Geometry: final body of the model. Coordinates: model frame, mm. A direction names the side the tool comes from. Coordinates: 2 decimals unless noted, no trailing zeros. Loops run counter-clockwise (first coordinate to the right, second up) from the corner with the lowest first, then second, coordinate; pieces in that order, holes last. Notation, with made-up numbers: (-1.5, 50.25) -> (28.5, 50.25) arc R25 ccw to (28.5, 74.25) -> close; hole circle Ø9 at (36, 34.25). An arc over 180 degrees is marked (long way). One line per item, written item: value. Start each with the question number.
from build123d import *

# Parameters (mm, degrees)
SKETCH_1_W              = 180
SKETCH_1_H              = 125
EXTRUDE_1_DEPTH         = 25
SKETCH_2_W              = 130
SKETCH_2_H              = 125
EXTRUDE_2_DEPTH         = 39
SKETCH_3_R              = 10
CUT_EXTRUDE_1_DEPTH     = 12
SKETCH_4_R              = 10
CUT_EXTRUDE_2_DEPTH     = 12
SKETCH_6_R              = 10
CUT_EXTRUDE_3_DEPTH     = 12
SKETCH_7_R              = 10
CUT_EXTRUDE_4_DEPTH     = 12
SKETCH_9_R              = 6.5
CUT_EXTRUDE_6_DEPTH     = 13
SKETCH_10_R             = 6.5
CUT_EXTRUDE_7_DEPTH     = 13
SKETCH_11_R             = 6.5
CUT_EXTRUDE_8_DEPTH     = 13
SKETCH_12_R             = 6.5
CUT_EXTRUDE_9_DEPTH     = 13
HOLE_WIZARD_M12_1_D     = 10.2
HOLE_WIZARD_M12_1_DEPTH = 25
HOLE_WIZARD_M12_1_TIP   = 3.064389157
HOLE_WIZARD_M12_2_D     = 10.2
HOLE_WIZARD_M12_2_DEPTH = 25
HOLE_WIZARD_M12_2_TIP   = 3.064389157
HOLE_WIZARD_M12_3_D     = 10.2
HOLE_WIZARD_M12_3_DEPTH = 25
HOLE_WIZARD_M12_3_TIP   = 3.064389157
HOLE_WIZARD_M12_4_D     = 10.2
HOLE_WIZARD_M12_4_DEPTH = 25
HOLE_WIZARD_M12_4_TIP   = 3.064389157
SKETCH_23_R             = 10.65
CUT_EXTRUDE_12_DEPTH    = 2
HOLE_WIZARD_M12_5_D     = 10.2
HOLE_WIZARD_M12_5_DEPTH = 25
HOLE_WIZARD_M12_5_TIP   = 3.064389157
HOLE_WIZARD_M12_6_D     = 10.2
HOLE_WIZARD_M12_6_DEPTH = 25
HOLE_WIZARD_M12_6_TIP   = 3.064389157
HOLE_WIZARD_M12_7_D     = 10.2
HOLE_WIZARD_M12_7_DEPTH = 25
HOLE_WIZARD_M12_7_TIP   = 3.064389157
FILLET_7_R              = 1
FILLET_8_R              = 1
FILLET_10_R             = 1
SKETCH_33_R             = 10.65
CUT_EXTRUDE_13_DEPTH    = 1.97
SKETCH_36_R             = 11.5
CUT_EXTRUDE_15_DEPTH    = 2
M16X1_5_2_D             = 14.5
M16X1_5_2_DEPTH         = 14
M16X1_5_2_TIP           = 4.356239488
SKETCH_38_R             = 6
CUT_EXTRUDE_16_DEPTH    = 63.03
MM_1_D                  = 12
MM_1_DEPTH              = 33.63
MM_1_TIP                = 3.605163714
SKETCH_41_R             = 11.5
CUT_EXTRUDE_17_DEPTH    = 2
SKETCH_39_R             = 10.65
CUT_EXTRUDE_18_DEPTH    = 1.97
CUT_EXTRUDE_19_REACH    = 125
SKETCH_42_R             = 6
M16X1_5_3_D             = 14.5
M16X1_5_3_DEPTH         = 14
M16X1_5_3_TIP           = 4.356239488
FILLET_11_R             = 1


with BuildPart() as part:
    # 草图1 → 凸台-拉伸1 (new body)
    with BuildSketch(Plane(origin=(0, 0, 0), x_dir=(1, 0, 0), z_dir=(0, 1, 0))):
        Rectangle(SKETCH_1_W, SKETCH_1_H)
    extrude(amount=EXTRUDE_1_DEPTH)

    # 草图2 → 凸台-拉伸2 (add)
    with BuildSketch(Plane(origin=(0, 25, 0), x_dir=(1, 0, 0), z_dir=(0, 1, 0))):
        Rectangle(SKETCH_2_W, SKETCH_2_H)
    extrude(amount=EXTRUDE_2_DEPTH)

    # 草图3 → 切除-拉伸1 (cut)
    with BuildSketch(Plane(origin=(0, 25, 0), x_dir=(1, 0, 0), z_dir=(0, 1, 0))):
        with Locations((-78, 44.5)):
            Circle(SKETCH_3_R)
    extrude(amount=-CUT_EXTRUDE_1_DEPTH, mode=Mode.SUBTRACT)

    # 草图4 → 切除-拉伸2 (cut)
    with BuildSketch(Plane(origin=(0, 25, 0), x_dir=(1, 0, 0), z_dir=(0, 1, 0))):
        with Locations((78, 44.5)):
            Circle(SKETCH_4_R)
    extrude(amount=-CUT_EXTRUDE_2_DEPTH, mode=Mode.SUBTRACT)

    # 草图6 → 切除-拉伸3 (cut)
    with BuildSketch(Plane(origin=(0, 25, 0), x_dir=(1, 0, 0), z_dir=(0, 1, 0))):
        with Locations((-78, -44.5)):
            Circle(SKETCH_6_R)
    extrude(amount=-CUT_EXTRUDE_3_DEPTH, mode=Mode.SUBTRACT)

    # 草图7 → 切除-拉伸4 (cut)
    with BuildSketch(Plane(origin=(0, 25, 0), x_dir=(1, 0, 0), z_dir=(0, 1, 0))):
        with Locations((78, -44.5)):
            Circle(SKETCH_7_R)
    extrude(amount=-CUT_EXTRUDE_4_DEPTH, mode=Mode.SUBTRACT)

    # 草图9 → 切除-拉伸6 (cut)
    with BuildSketch(Plane(origin=(0, 13, 0), x_dir=(1, 0, 0), z_dir=(0, 1, 0))):
        with Locations((-78, -44.5)):
            Circle(SKETCH_9_R)
    extrude(amount=-CUT_EXTRUDE_6_DEPTH, mode=Mode.SUBTRACT)

    # 草图10 → 切除-拉伸7 (cut)
    with BuildSketch(Plane(origin=(0, 13, 0), x_dir=(1, 0, 0), z_dir=(0, 1, 0))):
        with Locations((-78, 44.5)):
            Circle(SKETCH_10_R)
    extrude(amount=-CUT_EXTRUDE_7_DEPTH, mode=Mode.SUBTRACT)

    # 草图11 → 切除-拉伸8 (cut)
    with BuildSketch(Plane(origin=(0, 13, 0), x_dir=(1, 0, 0), z_dir=(0, 1, 0))):
        with Locations((78, 44.5)):
            Circle(SKETCH_11_R)
    extrude(amount=-CUT_EXTRUDE_8_DEPTH, mode=Mode.SUBTRACT)

    # 草图12 → 切除-拉伸9 (cut)
    with BuildSketch(Plane(origin=(0, 13, 0), x_dir=(1, 0, 0), z_dir=(0, 1, 0))):
        with Locations((78, -44.5)):
            Circle(SKETCH_12_R)
    extrude(amount=-CUT_EXTRUDE_9_DEPTH, mode=Mode.SUBTRACT)

    # M12 螺纹孔1
    with Locations(Plane(origin=(0, 64, 0), x_dir=(1, 0, 0), z_dir=(0, 1, 0))):
        with Locations((-55, 52.5)):
            Hole(HOLE_WIZARD_M12_1_D / 2, depth=HOLE_WIZARD_M12_1_DEPTH)
            with Locations((0, 0, -(HOLE_WIZARD_M12_1_DEPTH + HOLE_WIZARD_M12_1_TIP / 2))):  # 118° drill point
                Cone(0, HOLE_WIZARD_M12_1_D / 2, HOLE_WIZARD_M12_1_TIP, mode=Mode.SUBTRACT)

    # M12 螺纹孔2
    with Locations(Plane(origin=(55, 64, -52.5), x_dir=(0, 0, 1), z_dir=(0, 1, 0))):
        with Locations((0, 0)):
            Hole(HOLE_WIZARD_M12_2_D / 2, depth=HOLE_WIZARD_M12_2_DEPTH)
            with Locations((0, 0, -(HOLE_WIZARD_M12_2_DEPTH + HOLE_WIZARD_M12_2_TIP / 2))):  # 118° drill point
                Cone(0, HOLE_WIZARD_M12_2_D / 2, HOLE_WIZARD_M12_2_TIP, mode=Mode.SUBTRACT)

    # M12 螺纹孔3
    with Locations(Plane(origin=(-55, 64, 52.5), x_dir=(0, 0, 1), z_dir=(0, 1, 0))):
        with Locations((0, 0)):
            Hole(HOLE_WIZARD_M12_3_D / 2, depth=HOLE_WIZARD_M12_3_DEPTH)
            with Locations((0, 0, -(HOLE_WIZARD_M12_3_DEPTH + HOLE_WIZARD_M12_3_TIP / 2))):  # 118° drill point
                Cone(0, HOLE_WIZARD_M12_3_D / 2, HOLE_WIZARD_M12_3_TIP, mode=Mode.SUBTRACT)

    # M12 螺纹孔4
    with Locations(Plane(origin=(55, 64, 52.5), x_dir=(0, 0, 1), z_dir=(0, 1, 0))):
        with Locations((0, 0)):
            Hole(HOLE_WIZARD_M12_4_D / 2, depth=HOLE_WIZARD_M12_4_DEPTH)
            with Locations((0, 0, -(HOLE_WIZARD_M12_4_DEPTH + HOLE_WIZARD_M12_4_TIP / 2))):  # 118° drill point
                Cone(0, HOLE_WIZARD_M12_4_D / 2, HOLE_WIZARD_M12_4_TIP, mode=Mode.SUBTRACT)

    # 草图23 → 切除-拉伸12 (cut)
    with BuildSketch(Plane.XZ):
        with Locations((-35, -27.5)):
            Circle(SKETCH_23_R)
    extrude(amount=-CUT_EXTRUDE_12_DEPTH, mode=Mode.SUBTRACT)

    # M12 螺纹孔5
    with Locations(Plane(origin=(55, 64, -52.5), x_dir=(0, 0, 1), z_dir=(0, 1, 0))):
        with Locations((0, 0)):
            Hole(HOLE_WIZARD_M12_5_D / 2, depth=HOLE_WIZARD_M12_5_DEPTH)
            with Locations((0, 0, -(HOLE_WIZARD_M12_5_DEPTH + HOLE_WIZARD_M12_5_TIP / 2))):  # 118° drill point
                Cone(0, HOLE_WIZARD_M12_5_D / 2, HOLE_WIZARD_M12_5_TIP, mode=Mode.SUBTRACT)

    # M12 螺纹孔6
    with Locations(Plane(origin=(-55, 64, 52.5), x_dir=(0, 0, 1), z_dir=(0, 1, 0))):
        with Locations((0, 0)):
            Hole(HOLE_WIZARD_M12_6_D / 2, depth=HOLE_WIZARD_M12_6_DEPTH)
            with Locations((0, 0, -(HOLE_WIZARD_M12_6_DEPTH + HOLE_WIZARD_M12_6_TIP / 2))):  # 118° drill point
                Cone(0, HOLE_WIZARD_M12_6_D / 2, HOLE_WIZARD_M12_6_TIP, mode=Mode.SUBTRACT)

    # M12 螺纹孔7
    with Locations(Plane(origin=(55, 64, 52.5), x_dir=(0, 0, 1), z_dir=(0, 1, 0))):
        with Locations((0, 0)):
            Hole(HOLE_WIZARD_M12_7_D / 2, depth=HOLE_WIZARD_M12_7_DEPTH)
            with Locations((0, 0, -(HOLE_WIZARD_M12_7_DEPTH + HOLE_WIZARD_M12_7_TIP / 2))):  # 118° drill point
                Cone(0, HOLE_WIZARD_M12_7_D / 2, HOLE_WIZARD_M12_7_TIP, mode=Mode.SUBTRACT)

    # 圆角7
    fillet_7_edges = [part.edges().sort_by_distance(p)[0] for p in [
        (-90, 25, 0),
    ]]
    fillet(fillet_7_edges, radius=FILLET_7_R)

    # 圆角8
    fillet_8_edges = [part.edges().sort_by_distance(p)[0] for p in [
        (-65, 25, 0),
    ]]
    fillet(fillet_8_edges, radius=FILLET_8_R)

    # 圆角10
    fillet_10_edges = [part.edges().sort_by_distance(p)[0] for p in [
        (65, 25, 0),
    ]]
    fillet(fillet_10_edges, radius=FILLET_10_R)

    # 草图33 → 切除-拉伸13 (cut)
    with BuildSketch(Plane(origin=(0, 64, 0), x_dir=(1, 0, 0), z_dir=(0, 1, 0))):
        with Locations((-35, 27.5)):
            Circle(SKETCH_33_R)
    extrude(amount=-CUT_EXTRUDE_13_DEPTH, mode=Mode.SUBTRACT)

    # 草图36 → 切除-拉伸15 (cut)
    with BuildSketch(Plane.XZ):
        with Locations((-35, -27.5)):
            Circle(SKETCH_36_R)
    extrude(amount=-CUT_EXTRUDE_15_DEPTH, mode=Mode.SUBTRACT)

    # M16x1.5 螺纹孔2
    with Locations(Plane(origin=(-35, 0, -27.5), x_dir=(0, 0, -1), z_dir=(0, -1, 0))):
        with Locations((0, 0)):
            Hole(M16X1_5_2_D / 2, depth=M16X1_5_2_DEPTH)
            with Locations((0, 0, -(M16X1_5_2_DEPTH + M16X1_5_2_TIP / 2))):  # 118° drill point
                Cone(0, M16X1_5_2_D / 2, M16X1_5_2_TIP, mode=Mode.SUBTRACT)

    # 草图38 → 切除-拉伸16 (cut, through all)
    with BuildSketch(Plane(origin=(0, 62.03, 0), x_dir=(1, 0, 0), z_dir=(0, 1, 0))):
        with Locations((-35, 27.5)):
            Circle(SKETCH_38_R)
    extrude(amount=-CUT_EXTRUDE_16_DEPTH, mode=Mode.SUBTRACT)

    # 大小mm 暗销孔1
    with Locations(Plane(origin=(5, 64, -7.5), x_dir=(0, 0, 1), z_dir=(0, 1, 0))):
        with Locations((0, 0)):
            Hole(MM_1_D / 2, depth=MM_1_DEPTH)
            with Locations((0, 0, -(MM_1_DEPTH + MM_1_TIP / 2))):  # 118° drill point
                Cone(0, MM_1_D / 2, MM_1_TIP, mode=Mode.SUBTRACT)

    # 草图41 → 切除-拉伸17 (cut)
    with BuildSketch(Plane.XY.offset(62.5)):
        with Locations((5, 35)):
            Circle(SKETCH_41_R)
    extrude(amount=-CUT_EXTRUDE_17_DEPTH, mode=Mode.SUBTRACT)

    # 草图39 → 切除-拉伸18 (cut)
    with BuildSketch(Plane(origin=(0, 64, 0), x_dir=(1, 0, 0), z_dir=(0, 1, 0))):
        with Locations((5, 7.5)):
            Circle(SKETCH_39_R)
    extrude(amount=-CUT_EXTRUDE_18_DEPTH, mode=Mode.SUBTRACT)

    # 草图42 → 切除-拉伸19 (cut, up to next)
    with BuildSketch(Plane.XY.offset(60.5), mode=Mode.PRIVATE) as cut_extrude_19_sk1:
        with Locations((5, 35)):
            Circle(SKETCH_42_R)
    cut_extrude_19_tool1 = extrude(cut_extrude_19_sk1.sketch, amount=-CUT_EXTRUDE_19_REACH, mode=Mode.PRIVATE) & part.part
    add(cut_extrude_19_tool1.solids().sort_by_distance((5, 35, 60.5))[0], mode=Mode.SUBTRACT)

    # M16x1.5 螺纹孔3
    with Locations(Plane(origin=(5, 35, 60.5), x_dir=(1, 0, 0), z_dir=(0, 0, 1))):
        with Locations((0, 0)):
            Hole(M16X1_5_3_D / 2, depth=M16X1_5_3_DEPTH)
            with Locations((0, 0, -(M16X1_5_3_DEPTH + M16X1_5_3_TIP / 2))):  # 118° drill point
                Cone(0, M16X1_5_3_D / 2, M16X1_5_3_TIP, mode=Mode.SUBTRACT)

    # 圆角11
    fillet_11_edges = [part.edges().sort_by_distance(p)[0] for p in [
        (90, 25, 0),
    ]]
    fillet(fillet_11_edges, radius=FILLET_11_R)


solid = part.part
1. Pin query (flat end, axial travel): pin 1 Ø6 at (y, z) = (45.5, 17.5) entering from -X; pin 2 Ø12 at (x, z) = (78, 44.5) entering from +Y; pin 3 Ø6.5 at (x, z) = (-38.5, -31) entering from +Y; pin 4 Ø9 at (x, z) = (55, -52.5) entering from +Y. Return the tip coordinate at first contact, or that it passes through.
2. Section C-C on x = -35. Return the cut outline in (y, z), plus the area to 3 significant figures.
3. Line query: L1, parallel to X at y = 6, z = 44; L2, parallel to Z at x = 78, y = 10.25; L3, parallel to X at y = 59, z = 52. Output: solid intervals per line, ascending. Write a range as [from, to].
4. Set-up query: faces 5 (the face through (-85.94, 19.08, -38.42)), 6 (the face through (90, 12, 1)), 7 (the face through (-4.126, 28.002, 61.514)), 8 (the face through (-39.412, 8.084, -33.253)). Return all of +Z, -Z, +X, -X, +Y, -Y with unobstructed straight access to the full face (end or side cutting, diameter ignored); none if empty.
5. Draft query along Z for faces 1 (the face through (-51.2, 51.3, -55.9)), 2 (the face through (-1, 32, -62.5)), 3 (the face through (-90, 12, 1)), 4 (the face through (-46.49, 0.99, -26.99)). Return one class per face: released by +Z, released by -Z, zero draft, split by the parting line, or undercut.
6. Section D-D on y = 19.5. Return the cut outline in (x, z).
7. Section B-B on x = 78. Return the cut outline in (y, z).
8. Section A-A on z = -44.5. Return the cut outline in (x, y).
Checks:
1. pin 1: x = -65
1. pin 2: through
1. pin 3: y = 62.03
1. pin 4: y = 38.64
2. outline: (0, -62.5) -> (64, -62.5) -> (64, -38.15) -> (62.03, -38.15) -> (62.03, -33.5) -> (14.75, -33.5) -> (14, -34.75) -> (2, -34.75) -> (2, -39) -> (0, -39) -> close; (0, -16) -> (2, -16) -> (2, -20.25) -> (14, -20.25) -> (14.75, -21.5) -> (62.03, -21.5) -> (62.03, -16.85) -> (64, -16.85) -> (64, 62.5) -> (0, 62.5) -> close
2. area: 7,160 mm²
3. L1: [-90, -84.48], [-71.52, 71.52], [84.48, 90]
3. L2: [-62.5, -51], [-38, 38], [51, 62.5]
3. L3: [-65, -60.08], [-49.92, 49.92], [60.08, 65]
4. face 5: +Y
4. face 6: +Z, -Z, +X, +Y, -Y
4. face 7: +Z
4. face 8: -Y
5. face 1: undercut
5. face 2: released by -Z
5. face 3: zero draft
5. face 4: undercut
6. outline: (-90, -62.5) -> (90, -62.5) -> (90, 62.5) -> (-90, 62.5) -> close; hole circle Ø20 at (-78, -44.5); hole circle Ø20 at (-78, 44.5); hole circle Ø12 at (-35, -27.5); hole circle Ø20 at (78, -44.5); hole circle Ø20 at (78, 44.5)
7. outline: (0, -62.5) -> (25, -62.5) -> (25, -54.5) -> (13, -54.5) -> (13, -51) -> (0, -51) -> close; (0, -38) -> (13, -38) -> (13, -34.5) -> (25, -34.5) -> (25, 34.5) -> (13, 34.5) -> (13, 38) -> (0, 38) -> close; (0, 51) -> (13, 51) -> (13, 54.5) -> (25, 54.5) -> (25, 62.5) -> (0, 62.5) -> close
8. outline: (-90, 0) -> (-84.5, 0) -> (-84.5, 13) -> (-88, 13) -> (-88, 25) -> (-89, 25) arc R1 ccw to (-90, 24) -> close; (-71.5, 0) -> (71.5, 0) -> (71.5, 13) -> (68, 13) -> (68, 25) -> (66, 25) arc R1 cw to (65, 26) -> (65, 64) -> (-65, 64) -> (-65, 26) arc R1 cw to (-66, 25) -> (-68, 25) -> (-68, 13) -> (-71.5, 13) -> close; (84.5, 0) -> (90, 0) -> (90, 24) arc R1 ccw to (89, 25) -> (88, 25) -> (88, 13) -> (84.5, 13) -> close
